The figure shows three views and two pictorial views of one solid part (mm, origin at its lowest corner). Answer the questions. A direction names the side the tool comes from. Round coordinates to 2 decimals unless told otherwise and drop trailing zeros. Order: outer loops, then holes, each group sorted by start corner. A loop starts at its lowest first (then second) coordinate and runs counter-clockwise, first axis right, second up. Notation, with made-up numbers: M 73.25,-9 L 96.25,-9 A30 cw 96.25,15 Z; hole C -7.75,-40 d3. An arc over 180 degrees is marked long. Answer as CSV lines item,"result".
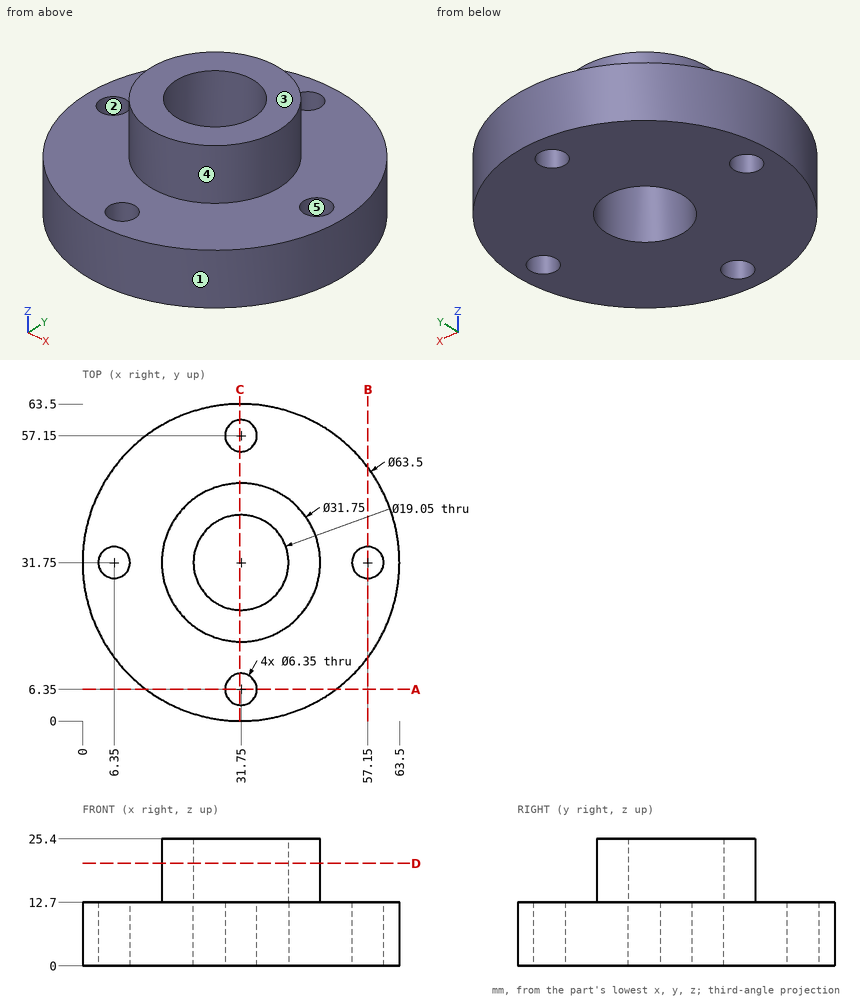
Item 1: Find the intervals of material crossed by probe 1 along Y at (x, z) = (31.75, 8.75) (3 decimals); probe 2 along X at (y, z) = (32, 16.75); probe 3 along Z at (x, y) = (47, 41.5), in increasing order. Write a range as [from, to].
Ans:
probe 1,"[0, 3.175], [9.525, 22.225], [41.275, 53.975], [60.325, 63.5]"
probe 2,"[15.88, 22.23], [41.27, 47.62]"
probe 3,"[0, 12.7]"
Item 2: A cutting plane is placed at D-D, the plane z = 20.5. Determine the outline of the cut face in (x, y) (3 decimals).
Ans:
outline,"C 31.75,31.75 d31.75; hole C 31.75,31.75 d19.05"
Item 3: A cutting plane is placed at C-C, the plane x = 31.5. Determine the outline of the cut face in (y, z).
Ans:
outline,"M 0,0 L 3.18,0 L 3.18,12.7 L 0,12.7 Z; M 9.52,0 L 22.23,0 L 22.23,25.4 L 15.88,25.4 L 15.88,12.7 L 9.52,12.7 Z; M 41.27,0 L 53.98,0 L 53.98,12.7 L 47.62,12.7 L 47.62,25.4 L 41.27,25.4 Z; M 60.32,0 L 63.5,0 L 63.5,12.7 L 60.32,12.7 Z"
Item 4: Flat-ended cylindrical pins translate along their axes: pin 1 (4 mm diameter, centred on x = 31.75, y = 6.35, fed in from +Z); pin 2 (6 mm diameter, centred on x = 43.5, z = 10, fed in from -Y); pin 3 (6 mm diameter, centred on y = 24.5, z = 8, fed in from -X); pin 4 (5 mm diameter, centred on x = 51.5, z = 14, fed in from -Y). Find the tip coordinate at first contact, or state that the pin passes through.
Ans:
pin 1,"through"
pin 2,"y = 1.23"
pin 3,"x = 0.29"
pin 4,"y = 5.33"
Item 5: A tool of negligible diameter and unlimited length cuts with its end or side. For the marked faces 4 and 5, from which of +Z, -Z, +X, -X, +Y, -Y can it reach the whole face along a straight path? Write none if from no direction.
Ans:
face 4,"+Z"
face 5,"+Z, -Z"
Item 6: Determine the mould class of the marked faces 1, 2 and 3 for opening direction X: +X half, -X half, draft (parallel to the pull), parting line (faces both ways), or undercut.
Ans:
face 1,"parting line"
face 2,"undercut"
face 3,"draft"
Item 7: A cutting plane is placed at A-A, the plane y = 6.35. Determine the outline of the cut face in (x, z) (3 decimals), and give its area (3 significant figures).
Ans:
outline,"M 12.7,0 L 28.575,0 L 28.575,12.7 L 12.7,12.7 Z; M 34.925,0 L 50.8,0 L 50.8,12.7 L 34.925,12.7 Z"
area,"403 mm2"
